Can you work these out from the model? Positions are in its coordinate system, mm. Face numbers are marked on the shaded views. A direction names the side the tool comes from. Coordinates: 2 decimals unless noted, no trailing zeros. Order: outer loops, then holes, each group sorted by start corner. A loop starts at its lowest first (then second) coordinate and runs counter-clockwise, first axis right, second up. Notation, with made-up numbers: (62.5, -26) -> (108.5, -26) arc R27 ccw to (108.5, 6) -> close; hole circle Ø6 at (66.25, 31.25). An arc over 180 degrees is marked (long way). Answer as a JSON object with one key per item and string values. Group by question number.
(1) Which directions (+Z, -Z, +X, -X, +Y, -Y) give clear straight access to the entire face, cutting with the end or side of a thin tool? Please do the marked faces 1, 2, 3, 4 and 5.
(2) For pin 1 (0.6 mm diameter, centred on x = -16, y = 21, fed in from -Z); pin 2 (4.5 mm diameter, centred on x = -17, y = 13, fed in from -Z); pin 3 (1.5 mm diameter, centred on x = -11.5, y = 3, fed in from -Z), each with a flat end and sliding along its axis, tell me the tip position at first contact or that it passes through.
(3) I want a section at A-A, the plane z = 26.5. List the corners of the cut face in (x, y) for me.
(4) I want a section at D-D, the plane y = 2. List the corners of the cut face in (x, z) for me, plus the area to 3 significant figures.
(5) If we mould it in two halves opening along Y, with no side actions, what happens to the marked faces 6, 7 and 8? For each: pulls with the +Y half, pulls with the -Y half, needs draft (parallel to the pull), parting line crosses it, or undercut.
(6) I need wall thicknesses on line 1 (Y direction, x = -9.75, z = 39.5); line 2 (Y direction, x = -10.75, z = 5); line 3 (X direction, y = 17.5, z = 20). Which ranges of each line are inside material? Lowest first, please.
(7) I want a section at B-B, the plane y = 19.25. List the corners of the cut face in (x, z) for me.
(8) I want a section at C-C, the plane x = -10.25. List the corners of the cut face in (y, z) for me, plus the area to 3 significant figures.
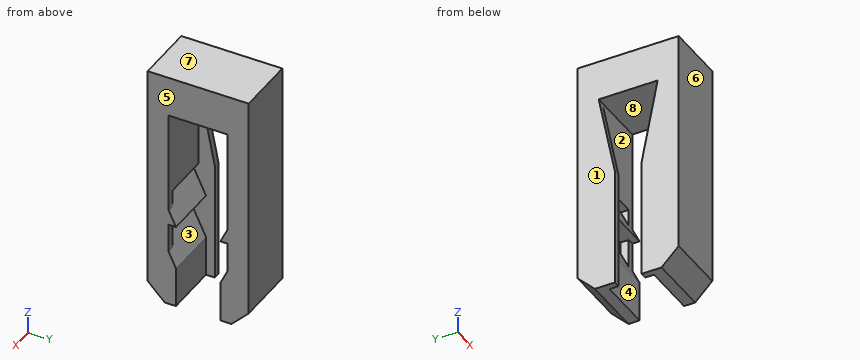
Autodesk Inventor part; units mm, degrees
ref_plane "YZ Plane" through (0, 0, 0) normal (1, 0, 0) x (0, 1, 0)
ref_plane "XZ Plane" through (0, 0, 0) normal (0, 1, 0) x (-1, 0, 0)
ref_plane "XY Plane" through (0, 0, 0) normal (0, 0, 1) x (1, 0, 0)
sketch "Эскиз1" plane through (0, 0, 0) normal (0, 1, 0) x (-1, 0, 0)
  line L0 (0, 0) -> (22, 0)
  line L1 (22, 0) -> (22, 60)
  line L2 (22, 60) -> (0, 60)
  line L3 (0, 60) -> (0, 0)
  dimension "d0" = 22
  dimension "d1" = 60
extrude "Выдавливание1" add sketch "Эскиз1" along normal blind 25
sketch "Эскиз2" plane through (0, 0, 60) normal (1, 0, 0) x (0, 0, -1)
  line L0 (60, 25) -> (0, 25)
  line L1 (60, 25) -> (60, 21.8)
  line L2 (60, 0) -> (60, 25)
  line L3 (60, 21.8) -> (20, 21.8)
  line L4 (60, 0) -> (0, 0)
  line L5 (60, 0) -> (60, 3.2)
  line L6 (60, 3.2) -> (20, 3.2)
  line L7 (20, 25) -> (20, 0)
  line L8 (20, 21.8) -> (28, 21.8)
  line L9 (20, 12.5) -> (60, 12.5)
  line L10 (60, 12.5) -> (60, 18)
  line L11 (60, 18) -> (13, 18)
  line L12 (28, 21.8) -> (28, 18)
  line L13 (28, 18) -> (20, 21.8)
  line L14 (28, 21.8) -> (31, 21.8)
  line L15 (31, 21.8) -> (39, 21.8)
  line L16 (39, 21.8) -> (39, 18)
  line L17 (39, 18) -> (31, 21.8)
  line L18 (39, 21.8) -> (42, 21.8)
  line L19 (42, 21.8) -> (50, 21.8)
  line L20 (50, 21.8) -> (50, 18)
  line L21 (42, 21.8) -> (50, 18)
  line L22 (20, 3.2) -> (28, 3.2)
  line L23 (28, 3.2) -> (28, 7)
  line L24 (28, 7) -> (20, 3.2)
  line L25 (31, 3.2) -> (39, 3.2)
  line L26 (39, 3.2) -> (39, 7)
  line L27 (39, 7) -> (31, 3.2)
  line L28 (42, 3.2) -> (50, 3.2)
  line L29 (50, 3.2) -> (50, 7)
  line L30 (42, 3.2) -> (50, 7)
  line L31 (50, 7) -> (63, 7)
  point P0 (22, 21.8)
  point P1 (60, 7)
  dimension "d4" = 3.2
  dimension "d5" = 3.2
  dimension "d6" = 40
  dimension "d7" = 5.5
  dimension "d8" = 8
  dimension "d9" = 8
  dimension "d10" = 3
  dimension "d11" = 8
extrude "Выдавливание2" cut sketch "Эскиз2" against normal through all contours L13 L11 L7 | L2 L9 L7 L11 | L3 L17 L11 L12 | L2 L31 L30 L6 L26 L27 L23 L24 L7 L9 | L11 L16 L3 L21
sketch "Эскиз3" plane through (0, 0, 60) normal (1, 0, 0) x (0, 0, -1)
  line L0 (50, 18) -> (60, 18)
  line L1 (60, 18) -> (60, 25)
  line L2 (0, 25) -> (60, 25)
  line L3 (0, 0) -> (0, 25)
  line L4 (0, 0) -> (60, 0)
  line L5 (60, 0) -> (60, 7)
  line L6 (60, 7) -> (50, 7)
  line L7 (50, 7) -> (42, 3.2)
  line L8 (42, 3.2) -> (39, 3.2)
  line L9 (39, 3.2) -> (39, 7)
  line L10 (39, 7) -> (31, 3.2)
  line L11 (31, 3.2) -> (28, 3.2)
  line L12 (28, 3.2) -> (28, 7)
  line L13 (28, 7) -> (20, 3.2)
  line L14 (20, 3.2) -> (20, 21.8)
  line L15 (20, 21.8) -> (28, 18)
  line L16 (28, 18) -> (28, 21.8)
  line L17 (28, 21.8) -> (31, 21.8)
  line L18 (31, 21.8) -> (39, 18)
  line L19 (39, 18) -> (39, 21.8)
  line L20 (39, 21.8) -> (42, 21.8)
  line L21 (42, 21.8) -> (50, 18)
chamfer "Фаска1" distance 4.25 angle 45 2 edges at (-11, 0, 0) (-11, 25, 0)
sketch "Эскиз4" plane through (0, 0, 60) normal (1, 0, 0) x (0, 0, -1)
  line L0 (20, 21.8) -> (28, 18)
  line L1 (20, 21.8) -> (31, 21.8)
  line L2 (31, 21.8) -> (31, 16.575)
  line L3 (31, 16.575) -> (20, 16.575)
  line L4 (20, 16.575) -> (20, 21.8)
  line L5 (20, 3.2) -> (20, 21.8)
  line L6 (20, 3.2) -> (30, 3.2)
  line L7 (30, 3.2) -> (30, 12)
  line L8 (30, 12) -> (20, 12)
  line L9 (20, 12) -> (20, 3.2)
  line L10 (20, 21.8) -> (10, 21.8)
  line L11 (10, 21.8) -> (10, 3.2)
  line L12 (10, 3.2) -> (20, 3.2)
  line L13 (20, 3.2) -> (20, 21.8)
  point P0 (60, 0)
extrude "Выдавливание3" cut sketch "Эскиз4" against normal through all
sketch "Эскиз5" plane through (0, 0, 60) normal (1, 0, 0) x (0, 0, -1)
  line L0 (31, 3.2) -> (10, 3.2)
  line L1 (10, 3.2) -> (10, 21.8)
  line L2 (10, 21.8) -> (31, 21.8)
  line L3 (31, 21.8) -> (39, 18)
  line L4 (39, 18) -> (39, 21.8)
  line L5 (39, 21.8) -> (42, 21.8)
  line L6 (42, 21.8) -> (50, 18)
  line L7 (50, 18) -> (60, 18)
  line L8 (60, 18) -> (60, 20.75)
  line L9 (55.75, 25) -> (60, 20.75)
  line L10 (0, 25) -> (55.75, 25)
  line L11 (0, 0) -> (0, 25)
  line L12 (0, 0) -> (55.75, 0)
  line L13 (60, 4.25) -> (55.75, 0)
  line L14 (60, 4.25) -> (60, 7)
  line L15 (60, 7) -> (50, 7)
  line L16 (50, 7) -> (42, 3.2)
  line L17 (42, 3.2) -> (39, 3.2)
  line L18 (39, 3.2) -> (39, 7)
  line L19 (39, 7) -> (31, 3.2)
  point P0 (60, 0)
extrude "Выдавливание4" cut sketch "Эскиз5" against normal blind 7
sketch "Эскиз6" plane through (-22, 0, 60) normal (-1, 0, 0) x (0, 0, 1)
  line L0 (-10, 21.8) -> (-10, 3.2)
  line L1 (-10, 3.2) -> (-10, 5.2)
  line L2 (-10, 5.2) -> (-31, 5.2)
  line L3 (-31, 5.2) -> (-31, 3.2)
  line L4 (-10, 3.2) -> (-31, 3.2)
  line L5 (-31, 3.2) -> (-39, 7)
  line L6 (-39, 7) -> (-39, 3.2)
  line L7 (-39, 3.2) -> (-42, 3.2)
  line L8 (-42, 3.2) -> (-50, 7)
  line L9 (-50, 7) -> (-60, 7)
  line L10 (-60, 4.25) -> (-60, 7)
  line L11 (-55.75, 0) -> (-60, 4.25)
  line L12 (-55.75, 0) -> (0, 0)
  line L13 (0, 0) -> (0, 25)
  line L14 (-55.75, 25) -> (0, 25)
  line L15 (-60, 20.75) -> (-55.75, 25)
  line L16 (-60, 18) -> (-60, 20.75)
  line L17 (-60, 18) -> (-50, 18)
  line L18 (-50, 18) -> (-42, 21.8)
  line L19 (-42, 21.8) -> (-39, 21.8)
  line L20 (-39, 21.8) -> (-39, 18)
  line L21 (-39, 18) -> (-31, 21.8)
  line L22 (-31, 21.8) -> (-10, 21.8)
  line L23 (-10, 21.8) -> (-10, 3.2)
  line L24 (-10, 21.8) -> (-31, 21.8)
  line L25 (-31, 21.8) -> (-31, 19.8)
  line L26 (-31, 19.8) -> (-10, 19.8)
  line L27 (-10, 19.8) -> (-10, 21.8)
  point P0 (-60, 0)
  point P1 (-31, 3.2)
  point P2 (-31, 21.8)
  dimension "d21" = 2
  dimension "d22" = 21
  dimension "d23" = 2
extrude "Выдавливание5" add sketch "Эскиз6" against normal up to surface (15 mm away) contours L0 L26 L25 L22 | L0 L4 L3 L2
sketch "Эскиз7" plane through (-22, 0, 60) normal (-1, 0, 0) x (0, 0, 1)
  line L0 (-10, 19.8) -> (-10, 5.2)
  line L1 (-10, 5.2) -> (-25, 5.2)
  line L2 (-25, 5.2) -> (-25, 9.2)
  line L3 (-25, 9.2) -> (-10, 9.2)
  line L4 (-10, 9.2) -> (-10, 5.2)
  line L5 (-10, 19.8) -> (-25, 19.8)
  line L6 (-25, 19.8) -> (-25, 15.8)
  line L7 (-25, 15.8) -> (-10, 15.8)
  line L8 (-10, 15.8) -> (-10, 19.8)
  line L9 (-31, 3.2) -> (-39, 7)
  line L10 (-39, 7) -> (-39, 3.2)
  line L11 (-39, 3.2) -> (-42, 3.2)
  line L12 (-42, 3.2) -> (-50, 7)
  line L13 (-50, 7) -> (-60, 7)
  line L14 (-60, 4.25) -> (-60, 7)
  line L15 (-55.75, 0) -> (-60, 4.25)
  line L16 (-55.75, 0) -> (0, 0)
  line L17 (0, 0) -> (0, 25)
  line L18 (-55.75, 25) -> (0, 25)
  line L19 (-60, 20.75) -> (-55.75, 25)
  line L20 (-60, 18) -> (-60, 20.75)
  line L21 (-60, 18) -> (-50, 18)
  line L22 (-50, 18) -> (-42, 21.8)
  line L23 (-42, 21.8) -> (-39, 21.8)
  line L24 (-39, 21.8) -> (-39, 18)
  line L25 (-39, 18) -> (-31, 21.8)
  line L26 (-31, 21.8) -> (-31, 19.8)
  line L27 (-31, 19.8) -> (-10, 19.8)
  line L28 (-10, 19.8) -> (-10, 5.2)
  line L29 (-10, 5.2) -> (-31, 5.2)
  line L30 (-31, 5.2) -> (-31, 3.2)
  line L31 (-60, 18) -> (-60, 7)
  line L32 (-25, 9.2) -> (-60, 9.2)
  line L33 (-25, 15.8) -> (-64.95, 15.8)
  line L34 (-30.4379, 9.2) -> (-10, 5.2)
  line L35 (-30.4379, 15.8) -> (-10, 19.8)
  point P0 (-60, 0)
  point P1 (-25, 19.8)
  point P2 (-25, 5.2)
  point P3 (-25, 5.2)
  point P4 (-60, 15.8)
  point P5 (-25, 19.8)
  dimension "d27" = 4
  dimension "d29" = 4
extrude "Выдавливание6" add sketch "Эскиз7" against normal blind 1.6 contours L35 L6 L5 | L6 L35 L33 L31 L21 L22 L23 L24 L25 L26 L27 | L1 L2 L34 | L29 L30 L9 L10 L11 L12 L13 L31 L32 L34 L2
sketch "Эскиз8" plane through (-7, 0, 60) normal (1, 0, 0) x (0, 0, -1)
  line L0 (31, 19.8) -> (72, 19.8)
  line L1 (31, 5.2) -> (69, 5.2)
  line L2 (50, 7) -> (60, 7)
  line L3 (42, 3.2) -> (50, 7)
  line L4 (39, 3.2) -> (42, 3.2)
  line L5 (39, 7) -> (39, 3.2)
  line L6 (31, 3.2) -> (39, 7)
  line L7 (31, 3.2) -> (31, 5.2)
  line L8 (31, 5.2) -> (10, 5.2)
  line L9 (10, 19.8) -> (10, 5.2)
  line L10 (10, 19.8) -> (31, 19.8)
  line L11 (31, 19.8) -> (31, 21.8)
  line L12 (39, 18) -> (31, 21.8)
  line L13 (39, 21.8) -> (39, 18)
  line L14 (42, 21.8) -> (39, 21.8)
  line L15 (50, 18) -> (42, 21.8)
  line L16 (60, 18) -> (50, 18)
  line L17 (60, 20.75) -> (60, 18)
  line L18 (55.75, 25) -> (60, 20.75)
  line L19 (0, 25) -> (55.75, 25)
  line L20 (0, 0) -> (0, 25)
  line L21 (55.75, 0) -> (0, 0)
  line L22 (60, 4.25) -> (55.75, 0)
  line L23 (60, 7) -> (60, 4.25)
  point P0 (60, 0)
  point P1 (46.2105, 5.2)
  point P2 (39, 5.2)
  point P3 (35.2105, 5.2)
  point P4 (35.2105, 19.8)
  point P5 (39, 19.8)
  point P6 (46.2105, 19.8)
extrude "Выдавливание7" add sketch "Эскиз8" against normal blind 1.6 contours L11 L12 L0 | L13 L14 L15 L0 | L1 L6 L7 | L1 L3 L4 L5
properties part number "встав для крюка"
Computed values:
{
 "1": {"face 1": "+Z, -Z, -X, +Y, -Y", "face 2": "+X", "face 3": "none", "face 4": "-Z, +X", "face 5": "+Z, -Z, +X, +Y, -Y"},
 "2": {"pin 1": "stops at z = 0", "pin 2": "stops at z = 50", "pin 3": "stops at z = 0.5"},
 "3": {"outline": "(-22, 0) -> (-7, 0) -> (-7, 5.2) -> (-8.6, 5.2) -> (-8.6, 4.39) -> (-20.4, 4.39) -> (-20.4, 9.2) -> (-22, 9.2) -> close; (-22, 15.8) -> (-20.4, 15.8) -> (-20.4, 20.61) -> (-8.6, 20.61) -> (-8.6, 19.8) -> (-7, 19.8) -> (-7, 25) -> (-22, 25) -> close"},
 "4": {"outline": "(-22, 2.25) -> (-7, 2.25) -> (-7, 60) -> (-22, 60) -> close", "area": "866 mm2"},
 "5": {"face 6": "pulls with the -Y half", "face 7": "needs draft", "face 8": "undercut"},
 "6": {"line 1": "y = 0 to 5.2, 19.8 to 25", "line 2": "y = 0 to 7, 18 to 25", "line 3": "x = -22 to -20.4"},
 "7": {"outline": "(-22, 0) -> (-7, 0) -> (-7, 12.63) -> (-20.4, 12.63) -> (-20.4, 21) -> (-7, 21) -> (-7, 23.63) -> (-20.4, 23.63) -> (-20.4, 47.19) -> (-22, 47.19) -> close; (-22, 50) -> (-7, 50) -> (-7, 60) -> (-22, 60) -> close"},
 "8": {"outline": "(0, 4.25) -> (4.25, 0) -> (7, 0) -> (7, 10) -> (3.2, 18) -> (3.2, 21) -> (7, 21) -> (3.2, 29) -> (5.2, 29) -> (5.2, 50) -> (19.8, 50) -> (19.8, 29) -> (21.8, 29) -> (18, 21) -> (21.8, 21) -> (21.8, 18) -> (18, 10) -> (18, 0) -> (20.75, 0) -> (25, 4.25) -> (25, 60) -> (0, 60) -> close", "area": "773 mm2"}
}
